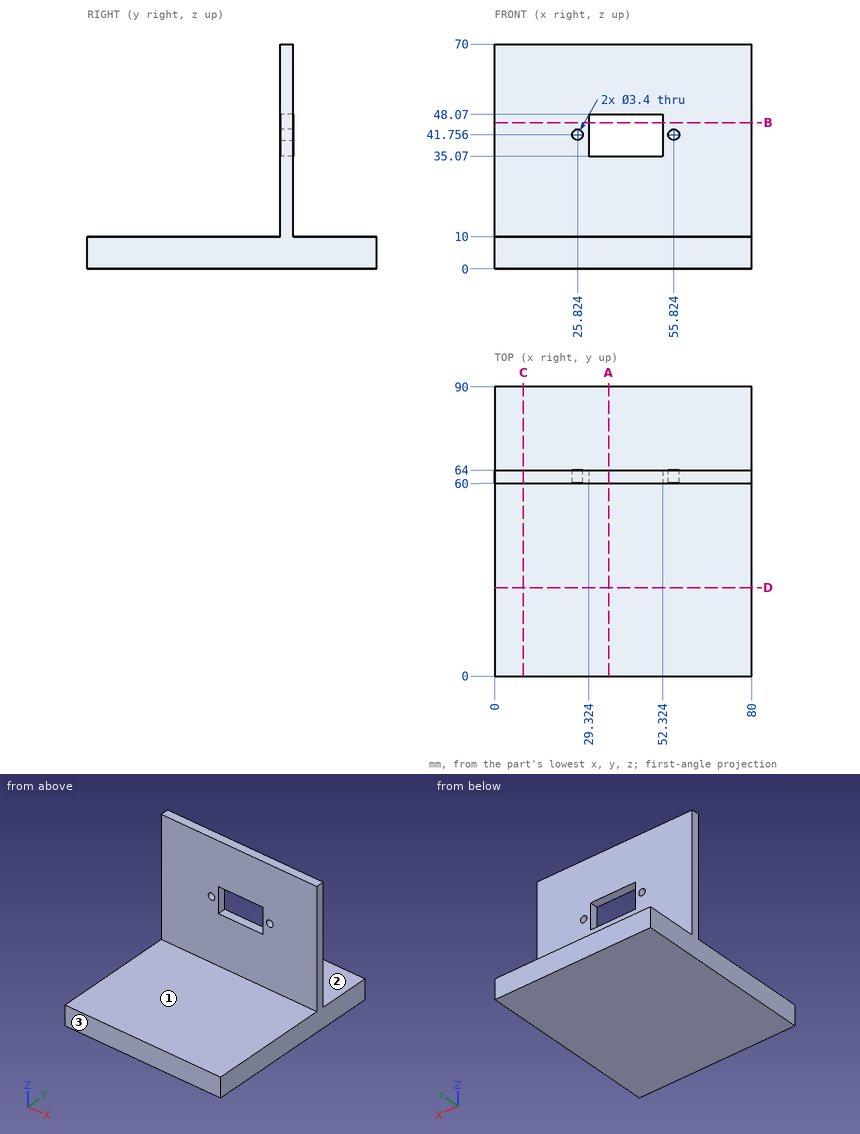
Design review of the part shown in the three views and the two pictorial views. Dimensions are in mm from the part's minimum x, y and z. A direction names the side the tool comes from. Coordinates: 2 decimals unless noted, no trailing zeros. Loops run counter-clockwise (first coordinate to the right, second up) from the corner with the lowest first, then second, coordinate; pieces in that order, holes last.
Q1. We need section B-B on z = 45.5. State the section outline as (x, y) points (1 decimal), and give its area (3 significant figures).
Reported:
outline: (0, 60) - (29.3, 60) - (29.3, 64) - (0, 64) - close; (52.3, 60) - (80, 60) - (80, 64) - (52.3, 64) - close
area: 228 mm2
Q2. For pin 1 (2 mm diameter, centred on x = 64.5, z = 41.5, fed in from +Y); pin 2 (1 mm diameter, centred on x = 41.5, y = 67, fed in from +Z); pin 3 (2 mm diameter, centred on x = 55.82, z = 41.76, fed in from -Y), all flat-tipped, find the tip position at first contact; note any pin that passes through.
Reported:
pin 1: stops at y = 64
pin 2: stops at z = 10
pin 3: passes through
Q3. We need section D-D on y = 27.5. State the section outline as (x, z) points.
Reported:
outline: (0, 0) - (80, 0) - (80, 10) - (0, 10) - close
Q4. To check wall thickness, follow line 1 (Y direction, x = 9.5, z = 48); line 2 (Z direction, x = 9, y = 66.5). State the ranges of each line that lie inside material, in increasing order.
Reported:
line 1: y = 60 to 64
line 2: z = 0 to 10
Q5. We need section C-C on x = 9. State the section outline as (y, z) points.
Reported:
outline: (0, 0) - (90, 0) - (90, 10) - (64, 10) - (64, 70) - (60, 70) - (60, 10) - (0, 10) - close
Q6. We need section A-A on x = 35.5. State the section outline as (y, z) points.
Reported:
outline: (0, 0) - (90, 0) - (90, 10) - (64, 10) - (64, 35.07) - (60, 35.07) - (60, 10) - (0, 10) - close; (60, 48.07) - (64, 48.07) - (64, 70) - (60, 70) - close
Q7. Tool access review of the marked faces 1, 2 and 3: name each direction out of +Z, -Z, +X, -X, +Y, -Y from which nothing blocks a thin tool from reaching the whole face with its end or side.
Reported:
face 1: +Z, +X, -X, -Y
face 2: +Z, +X, -X, +Y
face 3: +Z, -Z, +X, -X, -Y
